```python
from build123d import *

# Parameters (mm, degrees)
F1_DEPTH = 6.35
F2_R     = 5.08
F3_R     = 1.778


with BuildPart() as f1:
    # F0 (on Top) → F1 (new body)
    with BuildSketch(Plane.XY):
        Polygon((31.75, 0), (0, 45.72), (-31.75, 0), (-1.27, 0), (-1.27, 35.56), (1.27, 35.56), (1.27, 0), align=None)
    extrude(amount=F1_DEPTH)

    # F2
    f2_edges = [f1.edges().sort_by_distance(p)[0] for p in [
        (-1.27, 0, 3.175),
        (1.27, 0, 3.175),
    ]]
    fillet(f2_edges, radius=F2_R)

    # F3
    f3_edges = [f1.edges().sort_by_distance(p)[0] for p in [
        (0, 45.72, 3.175),
        (31.75, 0, 3.175),
        (-31.75, 0, 3.175),
    ]]
    fillet(f3_edges, radius=F3_R)


solid = f1.part
```
The listing builds one solid part. Answer for the finished solid, in the listing's coordinates (mm). A direction names the side the tool comes from. Round coordinates to 2 decimals unless told otherwise and drop trailing zeros. Loops run counter-clockwise (first coordinate to the right, second up) from the corner with the lowest first, then second, coordinate; pieces in that order, holes last. Notation, with made-up numbers: (15, 24) -> (69, 24) arc R17 ccw to (69, 38) -> close; hole circle Ø11 at (-14, 9). An arc over 180 degrees is marked (long way). Use one line per item in the form item = value.
1. The part is cut by section C-C on x = -18. Determine the outline of the cut face in (y, z).
Answer key:
outline = (0, 0) -> (19.8, 0) -> (19.8, 6.35) -> (0, 6.35) -> close
2. A tool of negligible diameter and unlimited length cuts with its end or side. For faces 5 (the flat face through (0, 35.56, 3)), 6 (the flat face through (-18, 0, 3)), from which of +Z, -Z, +X, -X, +Y, -Y can it reach the whole face along a straight path? Write none if from no direction.
Answer key:
face_5 = +Z, -Z, -Y
face_6 = +Z, -Z, +X, -X, -Y
3. Find the intervals of material crossed by probe 1 along X at (y, z) = (4.5, 4.5) (3 decimals); probe 2 along X at (y, z) = (22, 3.75); probe 3 along X at (y, z) = (42, 2.25), in increasing order. Write a range as [from, to].
Answer key:
probe_1 = [-28.625, -1.303], [1.303, 28.625]
probe_2 = [-16.47, -1.27], [1.27, 16.47]
probe_3 = [-2.58, 2.58]
4. For a pull along X with two mould halves and no side action, classify faces 1 (the flat face through (6, 13, 0)), 2 (the flat face through (-1.27, 20, 3)), 3 (the cylindrical face through (-2.798, 1.449, 3.219)), 4 (the cylindrical face through (-0.02, 44.38, 3.22)) as released by +X, released by -X, zero draft, split by the parting line, or undercut.
Answer key:
face_1 = zero draft
face_2 = undercut
face_3 = undercut
face_4 = split by the parting line
5. Flat-ended cylindrical pins translate along their axes: pin 1 Ø2 at (x, z) = (-5, 3) entering from +Y; pin 2 Ø1.5 at (y, z) = (33.5, 1) entering from +X. Find the tip coordinate at first contact, or state that the pin passes through.
Answer key:
pin_1 = 39.96
pin_2 = 9.01
6. The part is cut by section A-A on y = 10. Determine the outline of the cut face in (x, z), and give its area (3 significant figures).
Answer key:
outline = (-24.81, 0) -> (-1.27, 0) -> (-1.27, 6.35) -> (-24.81, 6.35) -> close; (1.27, 0) -> (24.81, 0) -> (24.81, 6.35) -> (1.27, 6.35) -> close
area = 299 mm²
7. The part is cut by section B-B on z = 2.25. Determine the outline of the cut face in (x, y), and give its area (3 significant figures).
Answer key:
outline = (-29.81, 2.79) arc R1.78 ccw to (-28.35, 0) -> (-6.35, 0) arc R5.08 ccw to (-1.27, 5.08) -> (-1.27, 35.56) -> (1.27, 35.56) -> (1.27, 5.08) arc R5.08 ccw to (6.35, 0) -> (28.35, 0) arc R1.78 ccw to (29.81, 2.79) -> (1.46, 43.62) arc R1.78 ccw to (-1.46, 43.62) -> close
area = 1,340 mm²
8. The part is cut by section D-D on y = 25.5. Determine the outline of the cut face in (x, z), and give its area (3 significant figures).
Answer key:
outline = (-14.04, 0) -> (-1.27, 0) -> (-1.27, 6.35) -> (-14.04, 6.35) -> close; (1.27, 0) -> (14.04, 0) -> (14.04, 6.35) -> (1.27, 6.35) -> close
area = 162 mm²
